```python
from build123d import *

# Parameters (mm, degrees)
F1_W          = 17.78
F1_H          = 17.78
F2_DEPTH      = 57.15
F4_SIZE       = 5.842
F6_W          = 8.255
F6_H          = 8.255
F7_DEPTH      = 57.15
F8_DEPTH      = 8.89
F10_T4_DEPTH  = 63.7100645368
F10_T9_DEPTH  = 63.7100645368
F10_T14_DEPTH = 15.4500645368
F10_T19_DEPTH = 63.7100645368
F10_T24_DEPTH = 63.7100645368
F10_T29_DEPTH = 15.4500645368
F12_W         = 11.43
F12_H         = 11.43
F13_DEPTH     = 57.15
F15_SIZE      = 3.81
F17_DEPTH     = 1.27
F19_DEPTH     = 1.905
F20_DEPTH     = 5.715
F21_T1_DEPTH  = 35.7625440314
F21_T6_DEPTH  = 35.7625440314
F21_T12_DEPTH = 35.7625440314
F21_T17_DEPTH = 35.7625440314
F21_T22_DEPTH = 35.7625440314
F22_DEPTH     = 1.5875
F25_DEPTH     = 7.0485


# Not quite as in the source:
# - a fillet or chamfer that OpenCascade refuses, or shapes differently, is made with other operations: its cross-section is extruded or revolved along the edge and cut away or added
# - an extrude ends at something that could not be found from the text; its depth is read off the source's solid


with BuildPart() as f2:
    # F1 (on Right) → F2 (new body)
    with BuildSketch(Plane.YZ):
        Rectangle(F1_W, F1_H)
    extrude(amount=F2_DEPTH)

    # F0 (on Front) → F3 (revolve, cut)
    with BuildSketch(Plane.XZ):
        Polygon((11.43, 3.175), (11.43, 0), (62.23, 0), (62.23, 6.35), (14.605, 6.35), align=None)
    revolve(axis=Axis((36.83, 0, 0), (1, 0, 0)), mode=Mode.SUBTRACT)

    # F4
    f4_edges = [f2.edges().sort_by_distance(p)[0] for p in [
        (28.575, -8.89, -8.89),
        (28.575, 8.89, 8.89),
        (28.575, -8.89, 8.89),
        (28.575, 8.89, -8.89),
    ]]
    chamfer(f4_edges, length=F4_SIZE)

    # F6 (on Top) → F7 (join)
    with BuildSketch(Plane.XY):
        Rectangle(F6_W, F6_H)
    extrude(amount=F7_DEPTH)

    # F8 (add, through all): a face of the model
    f8_faces = [f2.faces().sort_by_distance(p)[0] for p in [
        (-2.06375, 0, 0),
    ]]
    extrude(f8_faces, amount=F8_DEPTH)

    # F5 (on Right) → F9 (revolve, cut)
    with BuildSketch(Plane.YZ):
        Polygon((0, 66.04), (0, 11.43), (0.79375, 11.43), (1.5875, 12.22375), (1.5875, 66.04), align=None)
    revolve(axis=Axis((0, 0, 38.735), (0, 0, -1)), mode=Mode.SUBTRACT)

    # F10: chamfer of 2.794 on 4 edges, made by hand


with BuildPart() as f10_tool2:
    # F10_s3 → F10_t4 (new body)
    with BuildSketch(Plane.XY.offset(0.6252177316)):
        Polygon((4.1275, 1.3335), (1.3335, 4.1275), (4.1275, 4.1275), align=None)
    extrude(amount=F10_T4_DEPTH)

    split(bisect_by=Plane(origin=(0, 5.969, 5.969), x_dir=(1, 0, 0), z_dir=(0, 0.7071067812, 0.7071067812)), keep=Keep.TOP)


with BuildPart() as f2_1:
    add(f2.part)

    # F10_t1: cut F10_tool2
    add(f10_tool2.part, mode=Mode.SUBTRACT)


with BuildPart() as f10_tool7:
    # F10_s8 → F10_t9 (new body)
    with BuildSketch(Plane.XY.offset(0.6252177316)):
        Polygon((4.1275, 1.3335), (1.3335, 4.1275), (4.1275, 4.1275), align=None)
    extrude(amount=F10_T9_DEPTH)

    split(bisect_by=Plane.XY.offset(8.89), keep=Keep.TOP)


with BuildPart() as f2_2:
    add(f2_1.part)

    # F10_t6: cut F10_tool7
    add(f10_tool7.part, mode=Mode.SUBTRACT)


with BuildPart() as f10_tool12:
    # F10_s13 → F10_t14 (new body)
    with BuildSketch(Plane.XY.offset(-0.6252177316)):
        Polygon((-2.794, 4.1275), (0, 1.3335), (0, 4.1275), align=None)
    extrude(amount=-F10_T14_DEPTH)

    split(bisect_by=Plane(origin=(0, 5.969, -5.969), x_dir=(1, 0, 0), z_dir=(0, 0.7071067812, -0.7071067812)), keep=Keep.TOP)


with BuildPart() as f2_3:
    add(f2_2.part)

    # F10_t11: cut F10_tool12
    add(f10_tool12.part, mode=Mode.SUBTRACT)


with BuildPart() as f10_tool17:
    # F10_s18 → F10_t19 (new body)
    with BuildSketch(Plane.XY.offset(0.6252177316)):
        Polygon((1.3335, -4.1275), (4.1275, -1.3335), (4.1275, -4.1275), align=None)
    extrude(amount=F10_T19_DEPTH)

    split(bisect_by=Plane.XY.offset(8.89), keep=Keep.TOP)


with BuildPart() as f2_4:
    add(f2_3.part)

    # F10_t16: cut F10_tool17
    add(f10_tool17.part, mode=Mode.SUBTRACT)


with BuildPart() as f10_tool22:
    # F10_s23 → F10_t24 (new body)
    with BuildSketch(Plane.XY.offset(0.6252177316)):
        Polygon((1.3335, -4.1275), (4.1275, -1.3335), (4.1275, -4.1275), align=None)
    extrude(amount=F10_T24_DEPTH)

    split(bisect_by=Plane(origin=(0, -5.969, 5.969), x_dir=(1, 0, 0), z_dir=(0, -0.7071067812, 0.7071067812)), keep=Keep.TOP)


with BuildPart() as f2_5:
    add(f2_4.part)

    # F10_t21: cut F10_tool22
    add(f10_tool22.part, mode=Mode.SUBTRACT)


with BuildPart() as f10_tool27:
    # F10_s28 → F10_t29 (new body)
    with BuildSketch(Plane.XY.offset(-0.6252177316)):
        Polygon((-2.794, -4.1275), (0, -1.3335), (0, -4.1275), align=None)
    extrude(amount=-F10_T29_DEPTH)

    split(bisect_by=Plane(origin=(0, -5.969, -5.969), x_dir=(1, 0, 0), z_dir=(0, -0.7071067812, -0.7071067812)), keep=Keep.TOP)


with BuildPart() as f2_6:
    add(f2_5.part)

    # F10_t26: cut F10_tool27
    add(f10_tool27.part, mode=Mode.SUBTRACT)

    # F12 (on Front) → F13 (join)
    with BuildSketch(Plane.XZ):
        Rectangle(F12_W, F12_H)
    extrude(amount=-F13_DEPTH)

    # F11 (on Top) → F14 (revolve, cut)
    with BuildSketch(Plane.XY):
        Polygon((0, 66.04), (-3.175, 66.04), (-3.175, 13.0175), (-1.5875, 11.43), (0, 11.43), align=None)
    revolve(axis=Axis((0, 24.5966146997, 0), (0, 1, 0)), mode=Mode.SUBTRACT)

    # F15
    f15_edges = [f2_6.edges().sort_by_distance(p)[0] for p in [
        (5.715, 31.6865, 5.715),
        (5.715, 31.6865, -5.715),
        (-5.715, 28.575, -5.715),
    ]]
    chamfer(f15_edges, length=F15_SIZE)

    # F16 (on Front) → F17 (join, symmetric)
    with BuildSketch(Plane.XZ):
        Polygon((43.18, 8.89), (4.1275, 47.9425), (4.1275, 42.8625), (38.1, 8.89), align=None)
    extrude(amount=F17_DEPTH, both=True)

    # F18 (on Top) → F19 (join, symmetric)
    with BuildSketch(Plane.XY):
        Polygon((43.18, 8.89), (5.715, 46.355), (5.715, 41.275), (38.1, 8.89), align=None)
    extrude(amount=F19_DEPTH, both=True)

    # F1 (on Right) → F20 (join, through all)
    with BuildSketch(Plane.YZ):
        Rectangle(F1_W, F1_H)
    extrude(amount=-F20_DEPTH)

    # F21: chamfer of 5.842 on 4 edges, made by hand

    # F21_s2 → F21_t1 (cut)
    with BuildSketch(Plane.YZ.offset(-20.7387720157)):
        Polygon((-3.048, -8.89), (-8.89, -3.048), (-8.89, -8.89), align=None)
    extrude(amount=F21_T1_DEPTH, mode=Mode.SUBTRACT)


with BuildPart() as f21_tool4:
    # F21_s5 → F21_t6 (new body)
    with BuildSketch(Plane.YZ.offset(15.0237720157)):
        Polygon((3.048, 8.89), (8.89, 3.048), (8.89, 8.89), align=None)
    extrude(amount=-F21_T6_DEPTH)

    split(bisect_by=Plane.XZ.offset(-4.1275), keep=Keep.BOTTOM)

    split(bisect_by=Plane.XY.offset(5.715), keep=Keep.TOP)


with BuildPart() as f2_7:
    add(f2_6.part)

    # F21_t3: cut F21_tool4
    add(f21_tool4.part, mode=Mode.SUBTRACT)


with BuildPart() as f21_tool10:
    # F21_s11 → F21_t12 (new body)
    with BuildSketch(Plane.YZ.offset(15.0237720157)):
        Polygon((-3.048, 8.89), (-8.89, 3.048), (-8.89, 8.89), align=None)
    extrude(amount=-F21_T12_DEPTH)

    split(bisect_by=Plane.XZ.offset(4.1275), keep=Keep.TOP)


with BuildPart() as f2_8:
    add(f2_7.part)

    # F21_t9: cut F21_tool10
    add(f21_tool10.part, mode=Mode.SUBTRACT)


with BuildPart() as f21_tool15:
    # F21_s16 → F21_t17 (new body)
    with BuildSketch(Plane.YZ.offset(15.0237720157)):
        Polygon((3.048, -8.89), (8.89, -3.048), (8.89, -8.89), align=None)
    extrude(amount=-F21_T17_DEPTH)

    split(bisect_by=Plane.XY.offset(-5.715), keep=Keep.BOTTOM)


with BuildPart() as f2_9:
    add(f2_8.part)

    # F21_t14: cut F21_tool15
    add(f21_tool15.part, mode=Mode.SUBTRACT)


with BuildPart() as f21_tool20:
    # F21_s21 → F21_t22 (new body)
    with BuildSketch(Plane.YZ.offset(15.0237720157)):
        Polygon((3.048, -8.89), (8.89, -3.048), (8.89, -8.89), align=None)
    extrude(amount=-F21_T22_DEPTH)

    split(bisect_by=Plane(origin=(-3.81, 0, -3.81), x_dir=(0, 1, 0), z_dir=(-0.7071067812, 0, -0.7071067812)), keep=Keep.TOP)


with BuildPart() as f2_10:
    add(f2_9.part)

    # F21_t19: cut F21_tool20
    add(f21_tool20.part, mode=Mode.SUBTRACT)

    # F22 (add, through all): a face of the model
    f22_faces = [f2_10.faces().sort_by_distance(p)[0] for p in [
        (-4.1275, 0, 33.02),
    ]]
    extrude(f22_faces, amount=F22_DEPTH)

    # F24 (on offset) → F25 (join, through all)
    with BuildSketch(Plane(origin=(-5.715, 0, 0), x_dir=(0, -1, 0), z_dir=(-1, 0, 0))):
        Polygon((-43.18, 5.715), (-38.1, 5.715), (-4.1275, 38.1), (-4.1275, 43.18), align=None)
    extrude(amount=-F25_DEPTH)


solid = f2_10.part
```
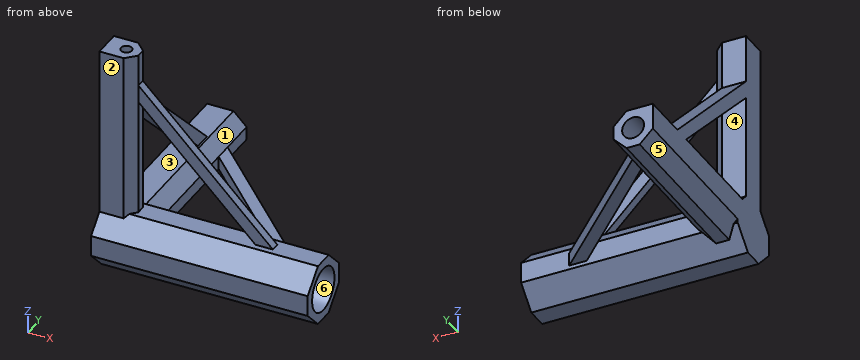
Here's how the part is built. I have some questions about the finished solid (model axes, mm). Face numbers are marked on the shaded views. A direction names the side the tool comes from. Give positions to 0.01 mm unless a question says otherwise; leave off trailing zeros. Write each loop counter-clockwise with the first axis right and the second up, starting at its lowest first coordinate (ties: lowest second). Pieces come first, ordered by that corner, then holes. Notation, with made-up numbers: (-1, 3.25) -> (6, 3.25) arc R23 cw to (6, 31.25) -> close; hole circle Ø8 at (32.25, 7.25). An arc over 180 degrees is marked (long way). Write each question's results on one line, items separated by ' | '.
Item 1: Suppose I cut it at D-D on x = 49. Write out the boundary of the cut face in (y, z).
Output:
outline: (-8.89, -3.05) -> (-3.05, -8.89) -> (3.05, -8.89) -> (8.89, -3.05) -> (8.89, 3.05) -> (3.05, 8.89) -> (-3.05, 8.89) -> (-8.89, 3.05) -> close; hole circle Ø12.7 at (0, 0)
Item 2: For pin 1 Ø2.5 at (x, y) = (-0.5, 27) entering from +Z; pin 2 Ø3.5 at (x, z) = (-2.5, 53.5) entering from +Y; pin 3 Ø8 at (y, z) = (0, 30) entering from +X, each with a flat end and sliding along its axis, tell me the tip position at first contact or that it passes through.
Output:
pin 1: stops at z = 22.44 | pin 2: stops at y = 4.13 | pin 3: stops at x = 26.07
Item 3: If I drill on L1, parallel to Y at x = 0, z = 21; L2, parallel to Y at x = 0, z = 33.5; L3, parallel to X at y = 0, z = 31 (1 decimal), over which ranges is the centre line in solid material (lowest first)?
Output:
L1: y = -4.13 to -1.59, 1.59 to 4.13, 22.07 to 27.25 | L2: y = -4.13 to -1.59, 1.59 to 4.13, 8.95 to 14.22 | L3: x = -5.7 to -1.6, 1.6 to 4.1, 16 to 21.1
Item 4: Suppose I cut it at A-A on x = 20. Write out the boundary of the cut face in (y, z) (3 decimals), plus the area to 3 significant figures.
Output:
outline: (-8.89, -3.048) -> (-3.048, -8.89) -> (3.048, -8.89) -> (8.89, -3.048) -> (8.89, 3.048) -> (3.048, 8.89) -> (-3.048, 8.89) -> (-8.89, 3.048) -> close; (-1.27, 26.99) -> (1.27, 26.99) -> (1.27, 32.07) -> (-1.27, 32.07) -> close; (26.99, -1.905) -> (32.07, -1.905) -> (32.07, 1.905) -> (26.99, 1.905) -> close; hole circle Ø12.7 at (0, 0) | area: 153 mm^2
Item 5: Suppose I cut it at C-C on y = 14.5. Give the number of separate pieces and of enclosed holes in the cut face, plus the area to 3 significant figures.
Output:
separate pieces: 3 | enclosed holes: 1 | area: 132 mm^2
Item 6: We'd pull the mould along Z, two halves only. Please class the marked faces 1, 2 and 3: pulls with the +Z half, pulls with the -Z half, needs draft (parallel to the pull), parting line crosses it, or undercut.
Output:
face 1: pulls with the +Z half | face 2: needs draft | face 3: undercut
Item 7: Suppose I cut it at B-B on z = 32. Write out the boundary of the cut face in (x, y) (1 decimal).
Output:
outline: (-5.7, -4.1) -> (1.3, -4.1) -> (4.1, -1.3) -> (4.1, 1.3) -> (1.3, 4.1) -> (-5.7, 4.1) -> close; (-5.7, 10.5) -> (1.3, 10.5) -> (1.3, 15.8) -> (-5.7, 15.8) -> close; (15, -1.3) -> (20.1, -1.3) -> (20.1, 1.3) -> (15, 1.3) -> close; hole circle Ø3.2 at (0, 0)
Item 8: On a 3-axis mill with a long thin cutter (end or side, diameter ignored), from which of +Z, -Z, +X, -X, +Y, -Y can I reach the whole of each face in a straight line? I mean the marked faces 4, 5 and 6. Say none if no direction works.
Output:
face 4: +X, -X | face 5: -Z, -X, +Y | face 6: +X
